Check sheet for the modelled part. Datum: model origin and axes. Units: mm. Face numbers are marked on the shaded views. A direction names the side the tool comes from. Round coordinates to 2 decimals unless told otherwise and drop trailing zeros. Order: outer loops, then holes, each group sorted by start corner. A loop starts at its lowest first (then second) coordinate and runs counter-clockwise, first axis right, second up. Notation, with made-up numbers: (72.25, 34) -> (128.25, 34) arc R7 cw to (128.25, 38) -> close; hole circle Ø9 at (88.5, 6.5). An arc over 180 degrees is marked (long way). Answer in a Markdown table with one row per item.
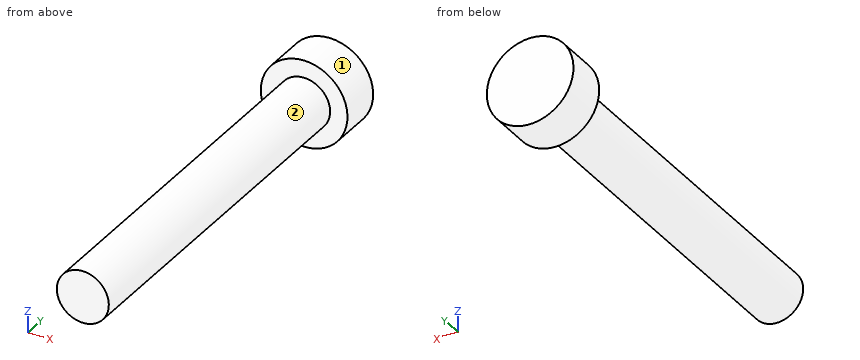
```python
from build123d import *

# Parameters (mm, degrees)
BOSS_EXTRUDE1_DEPTH      = 29.718
BOSS_EXTRUDE1_DEPTH_BACK = 8.89
SKETCH2_R                = 3.048
SKETCH3_R                = 5.08
BOSS_EXTRUDE2_DEPTH      = 5.08
SKETCH4_R                = 3.048
BOSS_EXTRUDE3_DEPTH      = 5.08


with BuildPart() as part:
    # Sketch2 → Boss-Extrude1 (new, two sides: drawn at the far end of the back side and taken through both)
    with BuildSketch(Plane(origin=(0, 0, 0), x_dir=(1, 0, 0), z_dir=(0, 1, 0)).offset(-BOSS_EXTRUDE1_DEPTH_BACK)):
        with Locations(Location((0, 0, 0), (0, 0, 270))):
            Circle(SKETCH2_R)
    extrude(amount=BOSS_EXTRUDE1_DEPTH + BOSS_EXTRUDE1_DEPTH_BACK)

    # Sketch3 → Boss-Extrude2 (add)
    with BuildSketch(Plane(origin=(0, 29.718, 0), x_dir=(1, 0, 0), z_dir=(0, 1, 0))):
        with Locations(Location((0, 0, 0), (0, 0, 270))):
            Circle(SKETCH3_R)
    extrude(amount=BOSS_EXTRUDE2_DEPTH)

    # Sketch4 → Boss-Extrude3 (add)
    with BuildSketch(Plane.XZ.offset(8.89)):
        with Locations(Location((0, 0, 0), (0, 0, 90))):
            Circle(SKETCH4_R)
    extrude(amount=BOSS_EXTRUDE3_DEPTH)


solid = part.part
```
(1) Section check D-D on y = 31.5. Record the boundary of the cut face in (x, z), plus the area to 3 significant figures.
Solutions:
| item | result |
|---|---|
| outline | circle Ø10.16 at (0, 0) |
| area | 81.1 mm^2 |
(2) Depth check by flat-ended pin: pin 1 Ø4 at (x, y) = (2.5, 0) entering from -Z; pin 2 Ø4 at (y, z) = (29.5, -4) entering from -X; pin 3 Ø2 at (y, z) = (14, -1) entering from -X. Enter the tip coordinate at first touch or a pass-through.
Solutions:
| item | result |
|---|---|
| pin 1 | z = -3.01 |
| pin 2 | x = -4.66 |
| pin 3 | x = -3.05 |
(3) Tool access check on the marked faces 1 and 2. Record the directions out of +Z, -Z, +X, -X, +Y, -Y that give a thin tool (end or side, any length) a straight path to the whole face; none if there is none.
Solutions:
| item | result |
|---|---|
| face 1 | +Y, -Y |
| face 2 | -Y |
(4) Section check C-C on y = 7.5. Record the boundary of the cut face in (x, z), plus the area to 3 significant figures.
Solutions:
| item | result |
|---|---|
| outline | circle Ø6.1 at (0, 0) |
| area | 29.2 mm^2 |
(5) Scan lines: probe 1 along Y at (x, z) = (-2.75, -2); probe 2 along Z at (x, y) = (-0.25, 19); probe 3 along X at (y, z) = (5.5, 0). Record each from-to range of solid material in increasing order. Write a range as from..to.
Solutions:
| item | result |
|---|---|
| probe 1 | 29.72..34.8 |
| probe 2 | -3.04..3.04 |
| probe 3 | -3.05..3.05 |
(6) Section check B-B on z = 0. Record the boundary of the cut face in (x, y).
Solutions:
| item | result |
|---|---|
| outline | (-5.08, 29.72) -> (-3.05, 29.72) -> (-3.05, -13.97) -> (3.05, -13.97) -> (3.05, 29.72) -> (5.08, 29.72) -> (5.08, 34.8) -> (-5.08, 34.8) -> close |
(7) Section check A-A on x = 0. Record the boundary of the cut face in (y, z), plus the area to 3 significant figures.
Solutions:
| item | result |
|---|---|
| outline | (-13.97, -3.05) -> (29.72, -3.05) -> (29.72, -5.08) -> (34.8, -5.08) -> (34.8, 5.08) -> (29.72, 5.08) -> (29.72, 3.05) -> (-13.97, 3.05) -> close |
| area | 318 mm^2 |
